Design review of the part built by this model. Coordinates are the model's own, in mm. A direction names the side the tool comes from. Round coordinates to 2 decimals unless told otherwise and drop trailing zeros. Order: outer loops, then holes, each group sorted by start corner. A loop starts at its lowest first (then second) coordinate and runs counter-clockwise, first axis right, second up. Notation, with made-up numbers: (-6.75, -38.5) - (23.25, -38.5) arc R16 cw to (23.25, -17.5) - close; hole circle Ø10 at (55, 25.25). An arc over 180 degrees is marked (long way). Use CSV: the item, a comma, the result in double quotes. Start each with the question number.
Autodesk Fusion 360 part; units mm, degrees
sketch "Sketch1" plane through (0, 0, 0) normal (0, 0, 1) x (1, 0, 0)
  circle A0 centre (0, 0) radius 15
extrude "Extrude1" add sketch "Sketch1" along normal blind 2
sketch "Sketch2" plane through (0, 0, 2) normal (0, 0, 1) x (-1, 0, 0)
  circle A0 centre (0, 0) radius 15
  circle A1 centre (0, -11) radius 1.5
  circle A2 centre (10.4616, -3.3992) radius 1.5
  circle A3 centre (6.4656, 8.8992) radius 1.5
  circle A4 centre (-6.4656, 8.8992) radius 1.5
  circle A5 centre (-10.4616, -3.3992) radius 1.5
  dimension "d4" = 360
extrude "Extrude2" cut sketch "Sketch2" against normal blind 19 contours A1 | A2 | A3 | A4 | A5
sketch "Sketch3" plane through (0, 0, 2) normal (0, 0, 1) x (-1, 0, 0)
  circle A0 centre (6.4656, 8.8992) radius 1.5
  circle A1 centre (10.4616, -3.3992) radius 1.5
  circle A2 centre (-6.4656, 8.8992) radius 1.5
  circle A3 centre (0, -11) radius 1.5
  circle A4 centre (-10.4616, -3.3992) radius 1.5
  circle A5 centre (0, 0) radius 15
  circle A6 centre (0, 0) radius 3
extrude "Extrude3" cut sketch "Sketch3" against normal blind 2 contours A6
sketch "Sketch4" plane through (0, 0, 2) normal (0, 0, 1) x (-1, 0, 0)
  circle A0 centre (0, 0) radius 3
  circle A1 centre (6.4656, 8.8992) radius 1.5
  circle A2 centre (10.4616, -3.3992) radius 1.5
  circle A3 centre (-6.4656, 8.8992) radius 1.5
  circle A4 centre (0, -11) radius 1.5
  circle A5 centre (-10.4616, -3.3992) radius 1.5
  circle A6 centre (0, 0) radius 15
  circle A7 centre (0, 0) radius 6.5
  dimension "d9" = 13
extrude "Extrude4" add sketch "Sketch4" along normal blind 9.5 contours A0 | A7
sketch "Sketch5" plane through (0, 0, 11.5) normal (0, 0, 1) x (-1, 0, 0)
  circle A0 centre (0, 0) radius 6.5
  circle A1 centre (0, 0) radius 4
extrude "Extrude5" add sketch "Sketch5" along normal blind 3.5 contours A1
sketch "Sketch6" plane through (0, 0, 2) normal (0, 0, -1) x (1, 0, 0)
  circle A0 centre (0, 0) radius 3
  circle A1 centre (0, 0) radius 1.5
  dimension "d14" = 3
extrude "Extrude6" cut sketch "Sketch6" against normal blind 100 contours A1
extrude "Extrude7" cut 1 faces at (-10.559, -3.3616, 0) along direction (0, 0, 1) blind 0.5
extrude "Extrude8" cut 1 faces at (-2.4832, 0.2236, 2) along direction (0, 0, 1) blind 0.5
Q1. Take a section at A-A (y = 0). State the section outline as (x, z) points, plus the area to 3 significant figures.
Q2. Clearance check with flat-ended pins moving along their axes: pin 1 (4 mm diameter, centred on x = 10.46, y = 3.4, fed in from +Z); pin 2 (1 mm diameter, centred on y = 0, z = 7.5, fed in from -X); pin 3 (1.8 mm diameter, centred on x = -10.46, y = 3.4, fed in from +Z); pin 4 (6 mm diameter, centred on x = 1.5, y = 9, fed in from +Z). State where each tip first meets the part, or that it passes through.
Q3. Take a section at B-B (x = -11.5). State the section outline as (y, z) points, plus the area to 3 significant figures.
Q4. For L1, parallel to X at y = 0, z = 7; L2, parallel to Z at x = -1.75, y = 0.75, list the stretches that pass through material, from the lowest coordinate up. Write a range as [from, to].
Q5. Take a section at D-D (x = 0.75). State the section outline as (y, z) points.
Q6. The part is to be moulded in two halves that separate along Y. For faces 1 (the flat face through (-3, -3, 11.5)), 2 (the cylindrical face through (0.867, -3.905, 13.226)), 3 (the cylindrical face through (0.325, 12.464, 1.26)), say which applies: +Y half, -Y half, draft (parallel to the pull), parting line (faces both ways), or undercut.
Q7. Take a section at C-C (z = 3). State the section outline as (x, y) points, plus the area to 3 significant figures.
Q8. Tool access review of faces 4 (the cylindrical face through (-8.963, 3.333, 1.26)), 5 (the flat face through (-1.3, 1.3, 2.5)), 6 (the cylindrical face through (5.158, -3.955, 6.684)): name each direction out of +Z, -Z, +X, -X, +Y, -Y from which nothing blocks a thin tool from reaching the whole face with its end or side.
Findings below:
1,outline,"(-15, 0.5) - (-3, 0.5) - (-3, 2.5) - (-1.5, 2.5) - (-1.5, 15) - (-4, 15) - (-4, 11.5) - (-6.5, 11.5) - (-6.5, 2) - (-15, 2) - close; (1.5, 2.5) - (3, 2.5) - (3, 0.5) - (15, 0.5) - (15, 2) - (6.5, 2) - (6.5, 11.5) - (4, 11.5) - (4, 15) - (1.5, 15) - close"
1,area,"147 mm^2"
2,pin 1,"stops at z = 2"
2,pin 2,"stops at x = -6.5"
2,pin 3,"passes through"
2,pin 4,"stops at z = 11.5"
3,outline,"(-9.63, 0.5) - (2.32, 0.5) - (2.32, 2) - (-9.63, 2) - close; (4.48, 0.5) - (9.63, 0.5) - (9.63, 2) - (4.48, 2) - close"
3,area,"25.6 mm^2"
4,L1,"x = [-6.5, -1.5], [1.5, 6.5]"
4,L2,"z = [2.5, 15]"
5,outline,"(-14.98, 0.5) - (-2.9, 0.5) - (-2.9, 2.5) - (-1.3, 2.5) - (-1.3, 15) - (-3.93, 15) - (-3.93, 11.5) - (-6.46, 11.5) - (-6.46, 2) - (-14.98, 2) - close; (1.3, 2.5) - (2.9, 2.5) - (2.9, 0.5) - (9.7, 0.5) - (9.7, 2) - (6.46, 2) - (6.46, 11.5) - (3.93, 11.5) - (3.93, 15) - (1.3, 15) - close; (12.3, 0.5) - (14.98, 0.5) - (14.98, 2) - (12.3, 2) - close"
6,face 1,"draft"
6,face 2,"parting line"
6,face 3,"undercut"
7,outline,"circle Ø13 at (0, 0); hole circle Ø3 at (0, 0)"
7,area,"126 mm^2"
8,face 4,"+Z, -Z"
8,face 5,"-Z"
8,face 6,"+Z"
